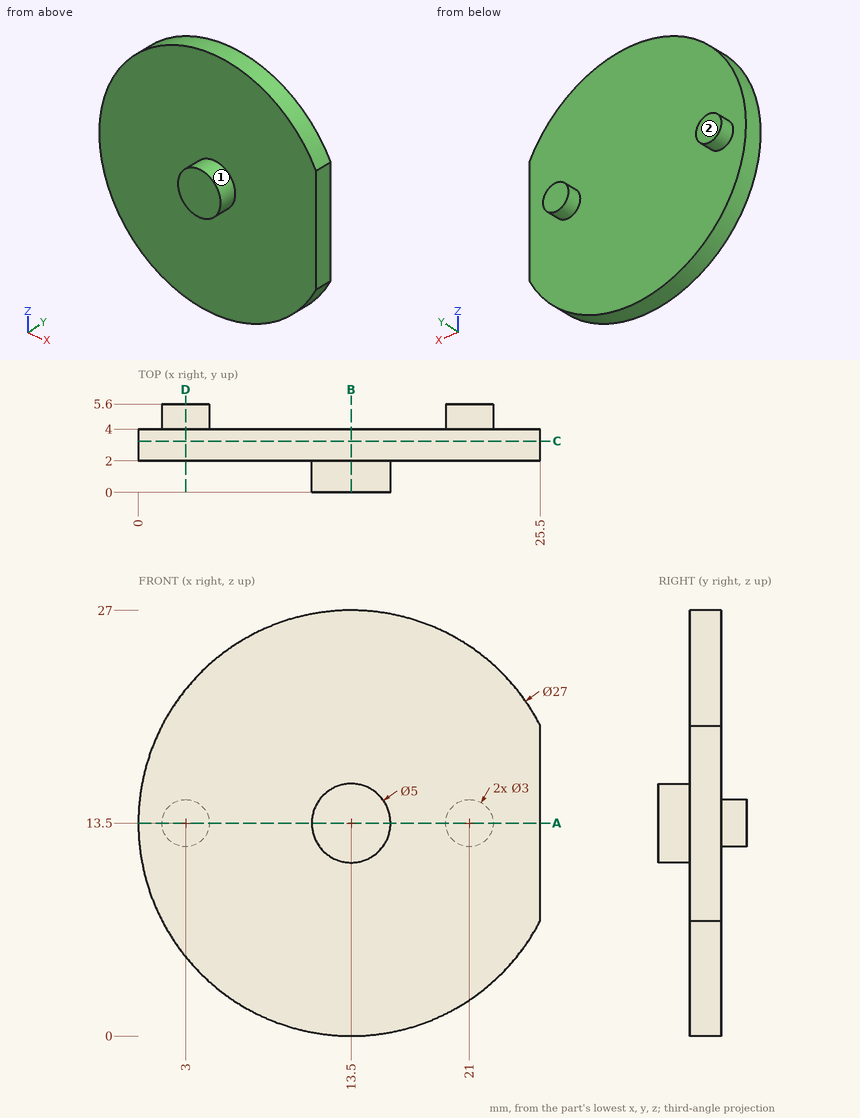
The figure shows three views and two pictorial views of one solid part (mm, origin at its lowest corner). Answer the questions. A direction names the side the tool comes from. Coordinates: 2 decimals unless noted, no trailing zeros. Write each loop counter-clockwise with the first axis right and the second up, starting at its lowest first coordinate (ties: lowest second). Pieces come first, ordered by that corner, then holes.
1. The part is cut by section C-C, the plane y = 3.25. Write down the section's boundary in (x, z), and give its area (3 significant figures).
Results list:
outline: (25.5, 7.32) - (25.5, 19.68) arc R13.5 ccw (long way) to start
area: 560 mm2
2. Consider line 1 along Y through (x, z) = (11, 6.5); line 2 along Y through (x, z) = (20.75, 13.25); line 3 along X through (y, z) = (2.05, 9.5). Determine where each line is inside the solid, lowest interval first.
Results list:
line 1: y = 2 to 4
line 2: y = 2 to 5.6
line 3: x = 0.61 to 25.5
3. The part is cut by section A-A, the plane z = 13.5. Write down the section's boundary in (x, y).
Results list:
outline: (0, 2) - (11, 2) - (11, 0) - (16, 0) - (16, 2) - (25.5, 2) - (25.5, 4) - (22.5, 4) - (22.5, 5.6) - (19.5, 5.6) - (19.5, 4) - (4.5, 4) - (4.5, 5.6) - (1.5, 5.6) - (1.5, 4) - (0, 4) - close
4. The part is cut by section B-B, the plane x = 13.5. Write down the section's boundary in (y, z).
Results list:
outline: (0, 11) - (2, 11) - (2, 0) - (4, 0) - (4, 27) - (2, 27) - (2, 16) - (0, 16) - close
5. The part is cut by section D-D, the plane x = 3. Write down the section's boundary in (y, z).
Results list:
outline: (2, 5.01) - (4, 5.01) - (4, 12) - (5.6, 12) - (5.6, 15) - (4, 15) - (4, 21.99) - (2, 21.99) - close
6. For the marked faces 1 and 2, determine the directions among +Z, -Z, +X, -X, +Y, -Y from which every point of the face is accessible in a straight line to the end or side of a thin tool.
Results list:
face 1: -Y
face 2: +Z, -Z, +X, -X, +Y
7. Flat-ended cylindrical pins translate along their axes: pin 1 (2 mm diameter, centred on x = 9, y = 3, fed in from -Z); pin 2 (4 mm diameter, centred on x = 8.5, z = 19.5, fed in from -Y); pin 3 (2 mm diameter, centred on x = 19.5, z = 7.5, fed in from +Y). Find the tip coordinate at first contact, or state that the pin passes through.
Results list:
pin 1: stops at z = 0.46
pin 2: stops at y = 2
pin 3: stops at y = 4
